Autodesk Fusion 360 part; units mm, degrees
sketch "Sketch1" plane through (0, 0, 0) normal (0, 0, 1) x (1, 0, 0)
  line L0 (0.0247, 50.0428) -> (30.0247, 50.0428)
  line L1 (30.0247, 50.0428) -> (30.0247, 25.0428)
  line L2 (30.0247, 25.0428) -> (0.0247, 25.0428)
  line L3 (0.0247, 25.0428) -> (0.0247, 50.0428)
  dimension "d3" = 30
  dimension "d4" = 25
extrude "Extrude1" add sketch "Sketch1" along normal blind 4
sketch "Sketch2" plane through (0, 0, 0) normal (0, 0, 1) x (1, 0, 0)
  line L0 (7.9626, 43.3083) -> (30.0026, 43.3083)
  line L1 (30.0026, 43.3083) -> (30.0026, 31.5625)
  line L2 (30.0026, 31.5625) -> (7.9626, 31.5625)
  line L3 (7.9626, 31.5625) -> (7.9626, 43.3083)
extrude "Extrude2" cut sketch "Sketch2" along normal blind 4
extrude "Extrude3" cut 1 faces at (30.0247, 41.7095, 1.3333) along direction (-1, 0, 0) blind 7
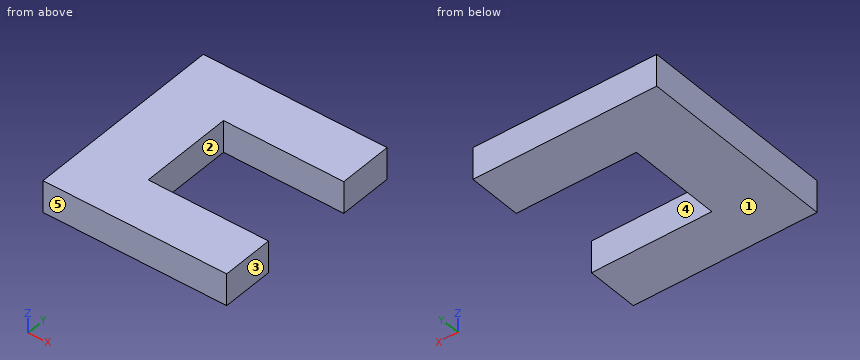
Source: CAD feature listing. Evaluate the final solid. Frame: model axes, mm. Face numbers are marked on the shaded views. A direction names the side the tool comes from. Coordinates: 2 decimals unless noted, no trailing zeros. Order: outer loops, then holes, each group sorted by start corner. A loop starts at its lowest first (then second) coordinate and runs counter-clockwise, first axis right, second up.
Item 1: Pull-direction query (Y, two-part tool) for the marked faces 3, 4 and 5; classes: pulls with the +Y half, pulls with the -Y half, needs draft (parallel to the pull), parting line crosses it, or undercut.
Output values:
face 3: needs draft
face 4: undercut
face 5: pulls with the -Y half
Item 2: Cut plane A-A (x = 16). Return loops of the section in (y, z), plus the area to 3 significant figures.
Output values:
outline: (25.04, 0) - (31.56, 0) - (31.56, 4) - (25.04, 4) - close; (43.31, 0) - (50.04, 0) - (50.04, 4) - (43.31, 4) - close
area: 53.0 mm2
Item 3: Material intervals for line 1 (Y direction, x = 21.5, z = 1.7); line 2 (X direction, y = 33.25, z = 1.2), sorted ascending.
Output values:
line 1: y = 25.04 to 31.56, 43.31 to 50.04
line 2: x = 0.02 to 7.96
Item 4: Cut plane B-B (z = 0.8). Return loops of the section in (x, y), plus the area to 3 significant figures.
Output values:
outline: (0.02, 25.04) - (23.02, 25.04) - (23.02, 31.56) - (7.96, 31.56) - (7.96, 43.31) - (23.02, 43.31) - (23.02, 50.04) - (0.02, 50.04) - close
area: 398 mm2
Item 5: Set-up query: the marked faces 1 and 2. Return all of +Z, -Z, +X, -X, +Y, -Y with unobstructed straight access to the full face (end or side cutting, diameter ignored); none if empty.
Output values:
face 1: -Z, +X, -X, +Y, -Y
face 2: +Z, -Z, +X
Item 6: Cut plane C-C (y = 34). Return loops of the section in (x, z), plus the area to 3 significant figures.
Output values:
outline: (0.02, 0) - (7.96, 0) - (7.96, 4) - (0.02, 4) - close
area: 31.8 mm2
Item 7: First-contact query: P1, Ø2, axis at y = 38, z = 1, coming from the +X side. Flat tip, straight axial feed; report the tip coordinate or a pass-through.
Output values:
P1: stops at x = 7.96
